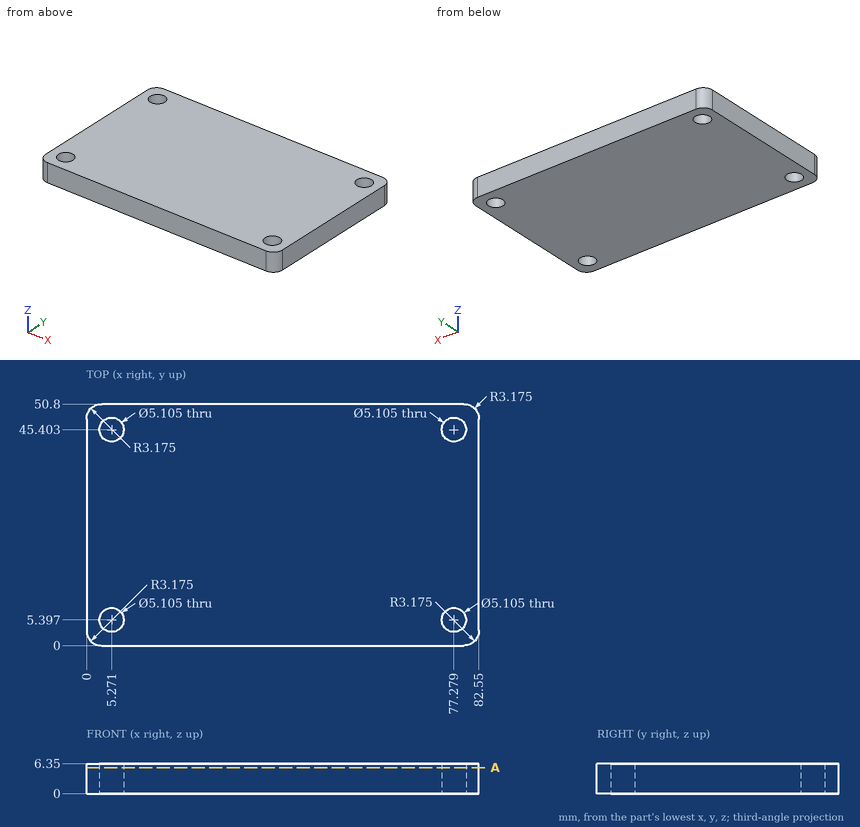
Check sheet for the drawn part. Datum: minimum x, y, z corner. Units: mm. Round coordinates to 2 decimals unless told otherwise and drop trailing zeros. Write item = value, one per line. Start each with the question number.
1. Depth check by flat-ended pin: pin 1 (6.5 mm diameter, centred on x = 77.28, y = 45.4, fed in from -Z); pin 2 (3 mm diameter, centred on x = 5.27, y = 5.4, fed in from +Z). Enter the tip coordinate at first touch or a pass-through.
2. Section check A-A on z = 5.5. Give the number of separate pieces and of enclosed holes in the cut face, then the cut area to 3 significant figures.
3. Thickness scan on line 1 (X direction, y = 45.5, z = 2.25); line 2 (Y direction, x = 7, z = 2.5) (1 decimal); line 3 (X direction, y = 45, z = 1.5). Record the ranges inside material, lowest first.
Working result:
q1.pin_1 = 0
q1.pin_2 = through
q2.separate_pieces = 1
q2.enclosed_holes = 4
q2.area = 4,100 mm^2
q3.line_1 = 0 to 2.72, 7.82 to 74.73, 79.83 to 82.55
q3.line_2 = 0 to 3.5, 7.3 to 43.5, 47.3 to 50.8
q3.line_3 = 0 to 2.75, 7.79 to 74.76, 79.8 to 82.55
